Autodesk Inventor part; units mm, degrees
ref_plane "YZ Plane" through (0, 0, 0) normal (1, 0, 0) x (0, 1, 0)
ref_plane "XZ Plane" through (0, 0, 0) normal (0, 1, 0) x (-1, 0, 0)
ref_plane "XY Plane" through (0, 0, 0) normal (0, 0, 1) x (1, 0, 0)
sketch "Sketch1" plane through (0, 0, 0) normal (0, 1, 0) x (-1, 0, 0)
  line L0 (0, 0) -> (16.8, 0)
  line L1 (16.8, 0) -> (16.8, -39)
  line L2 (16.8, -39) -> (0, -39)
  line L3 (0, -39) -> (0, 0)
  line L4 (16.8, -10.8) -> (10.7, -10.8)
  line L5 (10.7, -10.8) -> (10.7, -31)
  line L6 (10.7, -31) -> (16.8, -31)
  line L7 (16.8, -31) -> (16.8, -10.8)
  line L8 (0, -25.4905) -> (10.7, -25.4905)
  line L9 (10.7, -25.4905) -> (10.7, -14.3627)
  line L10 (10.7, -14.3627) -> (0, -14.3627)
  line L11 (0, -14.3627) -> (0, -25.4905)
  dimension "d0" = 16.8
  dimension "d1" = 39
  dimension "d2" = 6.1
  dimension "d3" = 20.2
  dimension "d4" = 0
  dimension "d5" = 10.7
  dimension "d6" = 8
extrude "Extrusion1" add sketch "Sketch1" along normal blind 1.6 contours L0 L1 L4 L5 L10 L3 | L10 L5 L8 L3 | L8 L5 L6 L1 L2 L3
extrude "Extrusion2" add sketch "Sketch1" along normal blind 2.4 and the other way blind 0.9 contours L1 L6 L5 L4
sketch "Sketch2" plane through (0, 2.4, 0) normal (0, 1, 0) x (1, 0, 0)
  line L0 (-16.95, 16.75) -> (-16.65, 16.75)
  line L1 (-15.65, 17.75) -> (-15.65, 24.05)
  line L2 (-16.65, 25.05) -> (-16.95, 25.05)
  line L3 (-17.95, 24.05) -> (-17.95, 17.75)
  line L4 (-16.8, 31) -> (-16.8, 10.8)
  line L5 (-10.7, 31) -> (-16.8, 31)
  line L6 (-16.8, 10.8) -> (-10.7, 10.8)
  arc A0 (-16.95, 25.05) -> (-17.95, 24.05) centre (-16.95, 24.05) ccw
  arc A1 (-15.65, 24.05) -> (-16.65, 25.05) centre (-16.65, 24.05) ccw
  arc A2 (-17.95, 17.75) -> (-16.95, 16.75) centre (-16.95, 17.75) ccw
  arc A3 (-16.65, 16.75) -> (-15.65, 17.75) centre (-16.65, 17.75) ccw
  point P0 (0, 0)
  point P1 (-17.95, 16.75)
  point P2 (-15.65, 25.05)
  point P3 (-17.95, 25.05)
  dimension "d13" = 2.3
  dimension "d14" = 8.3
  dimension "d15" = 1.15
  dimension "d16" = 5.95
  dimension "d17" = 5.95
  dimension "d18" = 1
extrude "Extrusion3" add sketch "Sketch2" along normal blind 11.4
sketch "Sketch3" plane through (0, 0, 0) normal (0, -1, 0) x (1, 0, 0)
  line L0 (0, 0) -> (0, -39)
  line L1 (0, 0) -> (-12, 0)
  line L2 (-12, 0) -> (-12, -10.8)
  line L3 (-12, -10.8) -> (0, -10.8)
  line L4 (0, -10.8) -> (0, 0)
  line L5 (-10.7, -31) -> (-16.8, -31)
  line L6 (-12, -31) -> (0, -31)
  line L7 (0, -31) -> (0, -39)
  line L8 (0, -39) -> (-12, -39)
  line L9 (-12, -39) -> (-12, -31)
  line L10 (-16.8, -39) -> (-12, -39)
  line L11 (-12, -39) -> (-12, -31)
  line L12 (-12, -31) -> (-16.8, -31)
  line L13 (-16.8, -31) -> (-16.8, -39)
  line L14 (-16.8, -10.8) -> (-12, -10.8)
  line L15 (-12, -10.8) -> (-12, 0)
  line L16 (-12, 0) -> (-16.8, 0)
  line L17 (-16.8, 0) -> (-16.8, -10.8)
  dimension "d21" = 12
  dimension "d22" = 10.8
extrude "Extrusion4" cut sketch "Sketch3" against normal blind 10.1 contours L2 L14 L17 L16 | L10 L13 L5 L9
sketch "Sketch4" plane through (0, 1.6, 0) normal (0, 1, 0) x (1, 0, 0)
  line L0 (0, 0) -> (0, 39)
  line L1 (0, 1.8) -> (-8.1, 1.8)
  line L2 (-8.1, 1.8) -> (-8.1, 9.3)
  line L3 (-8.1, 9.3) -> (0, 9.3)
  line L4 (0, 9.3) -> (0, 1.8)
  line L5 (-12, 0) -> (0, 0)
  point P0 (0, 9.3)
  dimension "d25" = 8.1
  dimension "d26" = 7.5
  dimension "d27" = 1.8
extrude "Extrusion5" add sketch "Sketch4" along normal blind 4
sketch "Sketch5" plane through (0, 0, 0) normal (1, 0, 0) x (0, 0, -1)
  line L0 (1.8, 5.6) -> (9.3, 5.6)
  line L1 (9.3, 1.6) -> (9.3, 5.6)
  line L2 (1.8, 5.6) -> (9.3, 5.6)
  line L3 (9.3, 5.6) -> (9.3, 1.6)
  line L4 (9.3, 1.6) -> (1.8, 1.6)
  line L5 (1.8, 1.6) -> (1.8, 5.6)
  point P0 (0, 0)
extrude "Extrusion6" add sketch "Sketch5" along normal blind 1
properties part number "eonPCB"
Source: CAD feature listing. Evaluate the final solid. Frame: model axes, mm. A direction names the side the tool comes from. Round coordinates to 2 decimals unless told otherwise and drop trailing zeros. Loops run counter-clockwise (first coordinate to the right, second up) from the corner with the lowest first, then second, coordinate; pieces in that order, holes last. Notation, with made-up numbers: M -11.5,-12 L 0.5,-12 A22 cw 0.5,20 Z; hole C 72.5,37.25 d2. An arc over 180 degrees is marked long. Use a Markdown table: item, result. Add a question column.
1. Cut plane C-C, the plane y = 12. Output: boundary loops of the cut face in (x, z), and give its area (3 significant figures).
2. Ray query, line 1 along Z through (x, y) = (-12.25, 1.75); line 2 along Y through (x, z) = (-8.25, -19.5); line 3 along Y through (x, z) = (-14.5, -22.5). Return the intervals inside material, ascending. Write a range as [from, to].
3. Cut plane A-A, the plane y = 4.25. Output: boundary loops of the cut face in (x, z).
4. Contact query for flat-ended pins moving along their axis: pin 1 (4.5 mm diameter, centred on x = -2.5, y = 3.5, fed in from -Z); pin 2 (1.3 mm diameter, centred on y = 0.5, z = -4.5, fed in from -X); pin 3 (6 mm diameter, centred on x = -9, y = 5.5, fed in from -Z); pin 4 (1.6 mm diameter, centred on x = -13, y = 0, fed in from +Z). Output: stop coordinate, or through.
5. Cut plane D-D, the plane z = -22.5. Output: boundary loops of the cut face in (x, y), and give its area (3 significant figures).
6. Cut plane B-B, the plane x = -3.5. Output: boundary loops of the cut face in (y, z), and give its area (3 significant figures).
7. Set-up query: faces 1 (the cylindrical face through (-15.951, 8.02, -24.765)), 2 (the flat face through (-15.65, 8, -21)), 3 (the flat face through (-8.1, 4, -5)). Return all of +Z, -Z, +X, -X, +Y, -Y with unobstructed straight access to the full face (end or side cutting, diameter ignored); none if empty.
Solution:
| question | item | result |
|---|---|---|
| 1 | outline | M -17.95,-24.05 A1 ccw -16.95,-25.05 L -16.65,-25.05 A1 ccw -15.65,-24.05 L -15.65,-17.75 A1 ccw -16.65,-16.75 L -16.95,-16.75 A1 ccw -17.95,-17.75 Z |
| 1 | area | 18.2 mm2 |
| 2 | line 1 | z = [-31, -10.8] |
| 2 | line 2 | y = [0, 1.6] |
| 2 | line 3 | y = [-0.9, 2.4] |
| 3 | outline | M -17.95,-24.05 A1 ccw -16.95,-25.05 L -16.65,-25.05 A1 ccw -15.65,-24.05 L -15.65,-17.75 A1 ccw -16.65,-16.75 L -16.95,-16.75 A1 ccw -17.95,-17.75 Z; M -8.1,-9.3 L 1,-9.3 L 1,-1.8 L -8.1,-1.8 Z |
| 4 | pin 1 | stops at z = -39 |
| 4 | pin 2 | stops at x = -12 |
| 4 | pin 3 | stops at z = -9.3 |
| 4 | pin 4 | stops at z = -10.8 |
| 5 | outline | M -17.95,2.4 L -16.8,2.4 L -16.8,-0.9 L -10.7,-0.9 L -10.7,0 L 0,0 L 0,1.6 L -10.7,1.6 L -10.7,2.4 L -15.65,2.4 L -15.65,13.8 L -17.95,13.8 Z |
| 5 | area | 63.5 mm2 |
| 6 | outline | M 0,-39 L 1.6,-39 L 1.6,-9.3 L 5.6,-9.3 L 5.6,-1.8 L 1.6,-1.8 L 1.6,0 L 0,0 Z |
| 6 | area | 92.4 mm2 |
| 7 | face 1 | -Z, +X, +Y |
| 7 | face 2 | +Z, -Z, +X, +Y |
| 7 | face 3 | +Z, -Z, -X, +Y |
